Here's the drawing with two shaded views (mm, measured from the low corner). I have some questions. A direction names the side the tool comes from. Give positions to 0.01 mm unless a question says otherwise; leave off trailing zeros. Write each loop counter-clockwise with the first axis right and the second up, starting at its lowest first coordinate (ties: lowest second). Pieces come first, ordered by that corner, then holes. Notation, with made-up numbers: (27.5, 83.25) - (49.5, 83.25) arc R28 ccw to (49.5, 121.25) - close; hole circle Ø6 at (-8, 3). An arc over 180 degrees is marked (long way). Answer as CSV lines item,"result". Start each with the question number.
Q1. Imagine slicing it at B-B on z = 12.7. State how many separate pieces and enclosed holes the cut face has, and give its area (3 significant figures).
Q2. Imagine slicing it at C-C on x = 48. List the corners of the cut face in (y, z) for me (1 decimal), and give its area (3 significant figures).
Q3. On a 3-axis mill with a long thin cutter (end or side, diameter ignored), from which of +Z, -Z, +X, -X, +Y, -Y can I reach the whole of each face in a straight line? I mean the marked faces 4, 5 and 6. Say none if no direction works.
Q4. We'd pull the mould along X, two halves only. Please class the marked faces 1, 2 and 3: pulls with the +X half, pulls with the -X half, needs draft (parallel to the pull), parting line crosses it, or undercut.
Q5. If I drill on line 1 along X through (y, z) = (1.85, 12.7) (1 decimal); line 2 along Y through (x, z) = (49.5, 56.5) (1 decimal); line 3 along Y through (x, z) = (6, 31.5), over which ranges is the centre line in solid material (lowest first)?
Q6. Will these pins go through, and if not, where does the flat tip stop? pin 1 Ø4 at (y, z) = (20, 53.5) entering from -X (1 decimal); pin 2 Ø10 at (y, z) = (19, 55) entering from +X; pin 3 Ø3 at (x, z) = (102.5, 29) entering from +Y.
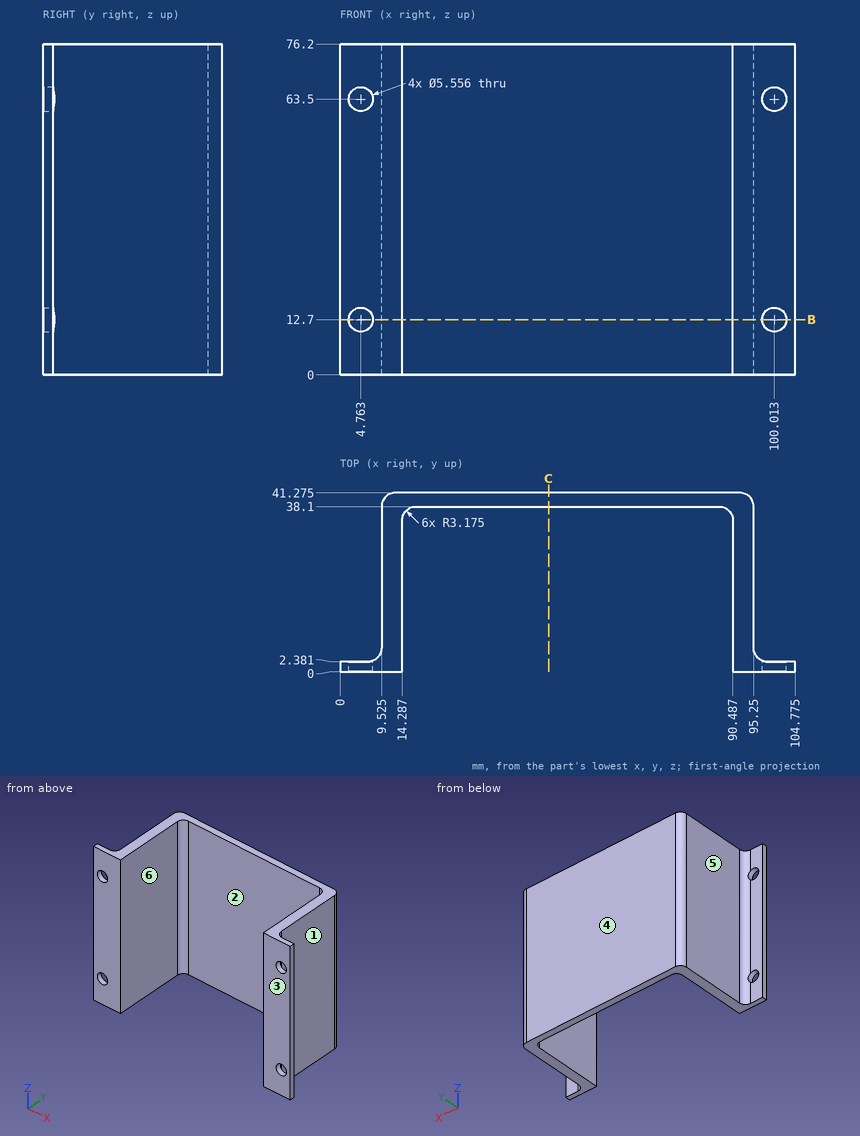
Conclusion:
1,separate pieces,"3"
1,enclosed holes,"0"
1,area,"658 mm^2"
2,outline,"(38.1, 0) - (41.3, 0) - (41.3, 76.2) - (38.1, 76.2) - close"
2,area,"242 mm^2"
3,face 4,"+Z, -Z, +X, -X, +Y"
3,face 5,"+Z, -Z, -X, +Y"
3,face 6,"+Z, -Z, -Y"
4,face 1,"pulls with the +X half"
4,face 2,"undercut"
4,face 3,"needs draft"
5,line 1,"0 to 2, 7.5 to 14.3, 90.5 to 97.2, 102.8 to 104.8"
5,line 2,"38.1 to 41.3"
5,line 3,"0 to 2.38"
6,pin 1,"x = 9.5"
6,pin 2,"x = 95.25"
6,pin 3,"y = 2.38"
